```python
from build123d import *

# Parameters (mm, degrees)
SKETCH_2_R               = 0.8
SKETCH_2_R_2             = 1
EXTRUDE_1_DEPTH          = 12
CUT_EXTRUDE_1_DEPTH      = 4
CUT_EXTRUDE_2_DEPTH      = 2
CUT_EXTRUDE_2_DEPTH_BACK = 2


with BuildPart() as part:
    # 草图2 → 凸台-拉伸1 (new body)
    with BuildSketch(Plane(origin=(0, 0, 0), x_dir=(1, 0, 0), z_dir=(0, 1, 0))):
        with BuildLine():
            Line((0, 0), (7, 0))
            ThreePointArc((7, 0), (8.5, -1.5), (7, -3))
            Line((7, -3), (0, -3))
            ThreePointArc((0, -3), (-1.5, -1.5), (0, 0))
        make_face()
        with Locations(Location((0, -1.5, 0), (0, 0, 270))):
            Circle(SKETCH_2_R, mode=Mode.SUBTRACT)
        with Locations(Location((7, -1.5, 0), (0, 0, 270))):
            Circle(SKETCH_2_R_2, mode=Mode.SUBTRACT)
    extrude(amount=EXTRUDE_1_DEPTH)

    # 草图4 → 切除-拉伸1 (cut)
    with BuildSketch(Plane.XZ):
        with BuildLine():
            Line((7, 0), (4, 0))
            ThreePointArc((4, 0), (5.5, 1.5), (4, 3))
            Line((4, 3), (7, 3))
            ThreePointArc((7, 3), (8.5, 1.5), (7, 0))
        make_face()
    cut_extrude_1 = extrude(amount=-CUT_EXTRUDE_1_DEPTH, mode=Mode.SUBTRACT)

    # 镜向1: 切除-拉伸1 across plane
    add(cut_extrude_1.mirror(Plane(origin=(0, 6, 0), x_dir=(0, 0, 1), z_dir=(0, -1, 0))), mode=Mode.SUBTRACT)

    # 草图5 → 切除-拉伸2 (cut, two sides: drawn at the far end of the back side and taken through both)
    with BuildSketch(Plane.XZ.offset(-6).offset(-CUT_EXTRUDE_2_DEPTH_BACK)):
        with BuildLine():
            Line((0, 3), (3, 3))
            ThreePointArc((3, 3), (1.5, 1.5), (3, 0))
            Line((3, 0), (0, 0))
            ThreePointArc((0, 0), (-1.5, 1.5), (0, 3))
        make_face()
    extrude(amount=CUT_EXTRUDE_2_DEPTH + CUT_EXTRUDE_2_DEPTH_BACK, mode=Mode.SUBTRACT)


solid = part.part
```
Input: part model. Units: mm. Frame: model coordinates. A direction names the side the tool comes from. Round coordinates to 2 decimals unless told otherwise and drop trailing zeros. Loops run counter-clockwise (first coordinate to the right, second up) from the corner with the lowest first, then second, coordinate; pieces in that order, holes last. Notation, with made-up numbers: (49, 45) -> (58, 45) arc R21 ccw to (58, 84) -> close; hole circle Ø7 at (-13.5, -40). An arc over 180 degrees is marked (long way). Use one line per item in the form item = value. Start each with the question number.
Item 1: Section query A-A on x = 1.25. Return the cut outline in (y, z).
Item 2: Mould query, pull axis Y, two halves, no side actions, for faces 4 (the face through (0, 10, 0.7)), 5 (the face through (1.5, 6, 1.5)), 6 (the face through (2, 12, 1)). Classes: pulls with the +Y half, pulls with the -Y half, needs draft (parallel to the pull), parting line crosses it, or undercut.
Item 3: Material intervals for L1, parallel to X at y = 6.85, z = 1.5; L2, parallel to Y at x = -1, z = 1.1; L3, parallel to X at y = 1.6, z = 1.5, sorted ascending. Write a range as from..to.
Item 4: Section query B-B on z = 1.5. Return the cut outline in (x, y), then the cut area to 3 significant figures.
Item 5: Section query C-C on y = 7.5. Return the cut outline in (x, z), then the cut area to 3 significant figures.
Item 6: Set-up query: faces 1 (the face through (2, 0, 1)), 2 (the face through (5.5, 2, 1.5)), 3 (the face through (5.5, 10, 1.5)). Return all of +Z, -Z, +X, -X, +Y, -Y with unobstructed straight access to the full face (end or side cutting, diameter ignored); none if empty.
Item 7: Contact query for flat-ended pins moving along their axis: pin 1 Ø2 at (x, y) = (1, 4) entering from -Z; pin 2 Ø1.5 at (x, z) = (6.5, 2) entering from -Y; pin 3 Ø1 at (y, z) = (6.5, 2.5) entering from -X; pin 4 Ø1 at (y, z) = (5.5, 1) entering from -X. Output: stop coordinate, or through.
Item 8: Section query D-D on x = -0.25. Return the cut outline in (y, z).
Ans:
q1.outline = (0, 0) -> (4, 0) -> (4, 3) -> (0, 3) -> close; (8, 0) -> (12, 0) -> (12, 3) -> (8, 3) -> close
q2.face_4 = needs draft
q2.face_5 = undercut
q2.face_6 = pulls with the +Y half
q3.L1 = 1.5..6, 8..8.5
q3.L2 = 0..4, 8..12
q3.L3 = -1.5..-0.8, 0.8..5.5
q4.outline = (-1.5, 0) -> (-0.8, 0) -> (-0.8, 4) -> (-1.5, 4) -> close; (-1.5, 8) -> (-0.8, 8) -> (-0.8, 12) -> (-1.5, 12) -> close; (0.8, 0) -> (5.5, 0) -> (5.5, 4) -> (6, 4) -> (6, 8) -> (5.5, 8) -> (5.5, 12) -> (0.8, 12) -> (0.8, 8) -> (1.5, 8) -> (1.5, 4) -> (0.8, 4) -> close; (8, 4) -> (8.5, 4) -> (8.5, 8) -> (8, 8) -> close
q4.area = 63.2 mm^2
q5.outline = (3, 0) -> (7, 0) arc R1.5 ccw to (7, 3) -> (3, 3) arc R1.5 ccw to start; hole circle Ø2 at (7, 1.5)
q5.area = 15.9 mm^2
q6.face_1 = +Z, -Z, +X, -X, -Y
q6.face_2 = +X, -Y
q6.face_3 = +X, +Y
q7.pin_1 = 0
q7.pin_2 = 4
q7.pin_3 = 1.59
q7.pin_4 = 1.5
q8.outline = (0, 0.02) -> (4, 0.02) -> (4, 0.74) -> (0, 0.74) -> close; (0, 2.26) -> (4, 2.26) -> (4, 2.98) -> (0, 2.98) -> close; (8, 0.02) -> (12, 0.02) -> (12, 0.74) -> (8, 0.74) -> close; (8, 2.26) -> (12, 2.26) -> (12, 2.98) -> (8, 2.98) -> close
